```python
from build123d import *

# Parameters (mm, degrees)
BOSS_EXTRUDE1_DEPTH      = 12.7
F_0000_CLEARANCE_HOLE1_D = 5.334
FILLET1_R                = 5.08
FILLET2_R                = 12.7


with BuildPart() as part:
    # Sketch1 → Boss-Extrude1 (new body)
    with BuildSketch(Plane.XY):
        Polygon((0, 0), (2.54, 0), (2.54, 31.75), (27.94, 31.75), (27.94, 0), (30.48, 0), (30.48, 34.29), (15.957826087, 34.29), (15.957826087, 68.58), (13.417826087, 68.58), (13.417826087, 34.29), (0, 34.29), align=None)
    extrude(amount=BOSS_EXTRUDE1_DEPTH)

    # #0000 Clearance Hole1 (through all)
    with Locations(Plane(origin=(0, 0, 0), x_dir=(0, 0, -1), z_dir=(-1, 0, 0))):
        with Locations((-6.35, -59.69), (-6.35, -8.89)):
            Hole(F_0000_CLEARANCE_HOLE1_D / 2)

    # Fillet1
    fillet1_edges = [part.edges().sort_by_distance(p)[0] for p in [
        (0, 34.29, 6.35),
        (30.48, 34.29, 6.35),
        (27.94, 31.75, 6.35),
        (2.54, 31.75, 6.35),
    ]]
    fillet(fillet1_edges, radius=FILLET1_R)

    # Fillet2
    fillet2_edges = [part.edges().sort_by_distance(p)[0] for p in [
        (14.687826087, 68.58, 0),
    ]]
    fillet(fillet2_edges, radius=FILLET2_R - 0.0001)  # a hair under: the kernel refuses the full size


solid = part.part
```
Geometry check sheet. Reference: the model listing, model coordinates, mm. A direction names the side the tool comes from. Coordinates: 2 decimals unless noted, no trailing zeros. Loops run counter-clockwise (first coordinate to the right, second up) from the corner with the lowest first, then second, coordinate; pieces in that order, holes last.
Item 1: Sectioned sample at C-C, the plane z = 5.25. Record the boundary of the cut face in (x, y).
Item 2: Go/stop test with flat-tipped pins: pin 1 Ø3 at (x, z) = (22.5, 8.5) entering from +Y; pin 2 Ø5 at (y, z) = (44, 4.5) entering from -X; pin 3 Ø4 at (x, z) = (13, 4) entering from -Y; pin 4 Ø4 at (y, z) = (8.5, 5.5) entering from -X. Record where each tip stops, or that it passes through.
Item 3: Thickness scan on line 1 (X direction, y = 16, z = 1.5); line 2 (Z direction, x = 1.2, y = 8.89); line 3 (X direction, y = 46.5, z = 4). Record the ranges inside material, lowest first.
Item 4: Access from +Z, -Z, +X, -X, +Y, -Y to the whole of each face (thin tool, end or side, straight path). Record for faces 4 (the face through (21, 34.29, 6)), 5 (the face through (3.989, 30.222, 6.439)), 6 (the face through (9, 34.29, 6)).
Item 5: Release check for a two-part mould opening along Z. For faces 1 (the face through (1.288, 11.256, 7.581)), 2 (the face through (15, 32, 0)), 3 (the face through (1.449, 32.762, 6.439)) record: released by +Z, released by -Z, zero draft, split by the parting line, or undercut.
Item 6: Sectioned sample at D-D, the plane x = 19. Record the boundary of the cut face in (y, z).
Item 7: Sectioned sample at A-A, the plane y = 18. Record the boundary of the cut face in (x, z), then the cut area to 3 significant figures.
Item 8: Sectioned sample at B-B, the plane y = 8.89. Record the boundary of the cut face in (x, z), then the cut area to 3 significant figures.
Check result:
1. outline: (0, 0) - (2.54, 0) - (2.54, 6.46) - (0, 6.46) - close; (0, 11.32) - (2.54, 11.32) - (2.54, 26.67) arc R5.08 cw to (7.62, 31.75) - (22.86, 31.75) arc R5.08 cw to (27.94, 26.67) - (27.94, 11.32) - (30.48, 11.32) - (30.48, 29.21) arc R5.08 ccw to (25.4, 34.29) - (15.96, 34.29) - (15.96, 57.26) - (13.42, 57.26) - (13.42, 34.29) - (5.08, 34.29) arc R5.08 ccw to (0, 29.21) - close; (13.42, 62.12) - (15.96, 62.12) - (15.96, 66.17) - (13.42, 66.17) - close; (27.94, 0) - (30.48, 0) - (30.48, 6.46) - (27.94, 6.46) - close
2. pin 1: stops at y = 34.29
2. pin 2: stops at x = 13.42
2. pin 3: stops at y = 31.75
2. pin 4: stops at x = 0
3. line 1: x = 0 to 2.54, 27.94 to 30.48
3. line 2: z = 0 to 3.68, 9.02 to 12.7
3. line 3: x = 13.42 to 15.96
4. face 4: +Z, -Z, +X, +Y
4. face 5: +Z, -Z, -Y
4. face 6: +Z, -Z, -X, +Y
5. face 1: undercut
5. face 2: released by -Z
5. face 3: zero draft
6. outline: (31.75, 0) - (34.29, 0) - (34.29, 12.7) - (31.75, 12.7) - close
7. outline: (0, 0) - (2.54, 0) - (2.54, 12.7) - (0, 12.7) - close; (27.94, 0) - (30.48, 0) - (30.48, 12.7) - (27.94, 12.7) - close
7. area: 64.5 mm2
8. outline: (0, 0) - (2.54, 0) - (2.54, 3.68) - (0, 3.68) - close; (0, 9.02) - (2.54, 9.02) - (2.54, 12.7) - (0, 12.7) - close; (27.94, 0) - (30.48, 0) - (30.48, 3.68) - (27.94, 3.68) - close; (27.94, 9.02) - (30.48, 9.02) - (30.48, 12.7) - (27.94, 12.7) - close
8. area: 37.4 mm2
